Could you check a few things on this model? Use its own coordinates, in mm. A direction names the side the tool comes from. Give positions to 0.01 mm unless a question says otherwise; leave off trailing zeros. Loops run counter-clockwise (first coordinate to the right, second up) from the corner with the lowest first, then second, coordinate; pieces in that order, holes last. Notation, with made-up numbers: (67, -30) -> (101, -30) arc R23 ccw to (101, 5) -> close; hole circle Ø2 at (17, 71). An arc over 180 degrees is marked (long way). Put each result on its own line as item: value.
```python
from build123d import *

# Parameters (mm, degrees)
F1_DEPTH = 31.75


with BuildPart() as f1:
    # F0 (on Top) → F1 (new body)
    with BuildSketch(Plane.XY):
        with BuildLine():
            Line((158.75, 260.35), (-158.75, 260.35))
            ThreePointArc((-158.75, 260.35), (-167.7302561211, 256.6302561211), (-171.45, 247.65))
            Line((-171.45, 247.65), (-171.45, -247.65))
            ThreePointArc((-171.45, -247.65), (-167.7302561211, -256.6302561211), (-158.75, -260.35))
            Line((-158.75, -260.35), (158.75, -260.35))
            ThreePointArc((158.75, -260.35), (167.7302561211, -256.6302561211), (171.45, -247.65))
            Line((171.45, -247.65), (171.45, 247.65))
            ThreePointArc((171.45, 247.65), (167.7302561211, 256.6302561211), (158.75, 260.35))
        make_face()
        with BuildLine():
            Line((-158.75, -168.3286130428), (-158.75, -69.85))
            add(Edge.make_bspline(
                [(-158.75, -69.85), (-125.750682879, -40.734982306), (-92.2382944115, 10.2020752056), (-121.6770256204, 92.6806720408), (-139.361128211, 110.4611489052)],
                knots=[0, 0, 0, 0, 0.5072023317, 1, 1, 1, 1], degree=3))
            Line((-139.361128211, 110.4611489052), (-139.361128211, 234.95))
            ThreePointArc((-139.361128211, 234.95), (-135.6413843321, 243.9302561211), (-126.661128211, 247.65))
            Line((-126.661128211, 247.65), (133.35, 247.65))
            ThreePointArc((133.35, 247.65), (142.3302561211, 243.9302561211), (146.05, 234.95))
            Line((146.05, 234.95), (146.05, 57.15))
            add(Edge.make_bspline(
                [(158.75, -103.9126433709), (142.5402943494, -66.7878627422), (75.9442820469, -25.835811925), (113.945925891, 34.7133202034), (146.05, 57.15)],
                knots=[0, 0, 0, 0, 0.5185201768, 1, 1, 1, 1], degree=3))
            add(Edge.make_bspline(
                [(0, -254), (66.0359377439, -253.8050247003), (118.9910289501, -216.3077578574), (171.45, -158.2672882658), (158.75, -103.9126433709)],
                knots=[0, 0, 0, 0, 0.5169156089, 1, 1, 1, 1], degree=3))
            add(Edge.make_bspline(
                [(0, -254), (-50.4826754374, -248.7984731698), (-144.7156709879, -239.3790961357), (-154.3932279359, -188.1159541937), (-158.75, -168.3286130428)],
                knots=[0, 0, 0, 0, 0.6026238082, 1, 1, 1, 1], degree=3))
        make_face(mode=Mode.SUBTRACT)
    extrude(amount=F1_DEPTH)


solid = f1.part
```
1. For faces 4 (the face through (167.83, 256.53, 15.65)), 5 (the face through (142.23, 244.03, 15.65)), which set-ups out of +Z, -Z, +X, -X, +Y, -Y let a thin tool reach every point of the face, with its end or its side?
Recorded:
face 4: +Z, -Z, +X, +Y
face 5: +Z, -Z
2. If we section it at A-A (y = 209.5): List the corners of the cut face in (x, z) for me.
Recorded:
outline: (-171.45, 0) -> (-139.36, 0) -> (-139.36, 31.75) -> (-171.45, 31.75) -> close; (146.05, 0) -> (171.45, 0) -> (171.45, 31.75) -> (146.05, 31.75) -> close
3. Thinking about a two-plate mould opening in Y: for faces 1 (the face through (171.45, -3, 16)), 2 (the face through (-158.75, -120, 16)), 3 (the face through (-167.63, 256.73, 15.65)), which applies, pulls with the +Y half, pulls with the -Y half, needs draft (parallel to the pull), parting line crosses it, or undercut?
Recorded:
face 1: needs draft
face 2: undercut
face 3: pulls with the +Y half
4. I need wall thicknesses on line 1 (X direction, y = 204.5, z = 28); line 2 (Y direction, x = 139, z = 25); line 3 (Y direction, x = -55, z = 2.5). Which ranges of each line are inside material? Lowest first, please.
Recorded:
line 1: x = -171.45 to -139.36, 146.05 to 171.45
line 2: y = -260.35 to -191.03, -72.36 to 51.94, 246.32 to 260.35
line 3: y = -260.35 to -247.55, 247.65 to 260.35
5. If we section it at B-B (x = 127): Count the separate pieces of the cut face and the enclosed holes in it, then the cut area to 3 significant figures.
Recorded:
separate pieces: 3
enclosed holes: 0
area: 5,370 mm^2
